from build123d import *

# Parameters (mm, degrees)
F0_R     = 60.254
F0_R_2   = 57.079
F1_DEPTH = 0.854
F2_R     = 60
F3_DEPTH = 0.6


with BuildPart() as f1:
    # F0 (on Top) → F1 (new body, symmetric)
    with BuildSketch(Plane.XY):
        Circle(F0_R)
        Circle(F0_R_2, mode=Mode.SUBTRACT)
    extrude(amount=F1_DEPTH, both=True)

    # F2 (on Top) → F3 (cut, symmetric)
    with BuildSketch(Plane.XY):
        Circle(F2_R)
    extrude(amount=F3_DEPTH, both=True, mode=Mode.SUBTRACT)


solid = f1.part
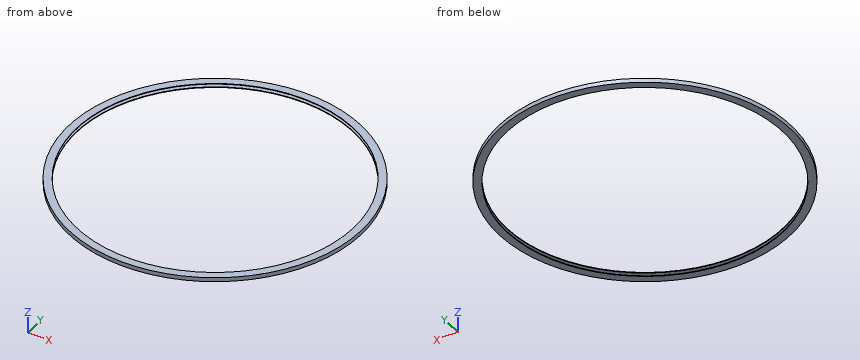
Source: CAD feature listing. Evaluate the final solid. Frame: model axes, mm. Coordinates: 2 decimals unless noted, no trailing zeros. Loops run counter-clockwise (first coordinate to the right, second up) from the corner with the lowest first, then second, coordinate; pieces in that order, holes last. Notation, with made-up numbers: (-8.75, 77.25) - (37.25, 77.25) arc R13 cw to (37.25, 87.25) - close; hole circle Ø3 at (87, 51.25). An arc over 180 degrees is marked (long way). One line per item, written item: value. Start each with the question number.
1. Contact query for a flat-ended pin moving along its axis: P1, Ø12, axis at x = -10.5, y = 46, coming from the +Z side. Output: stop coordinate, or through.
2. Section C-C (z = -0.15). Return the cut outline in (x, y), and give its area (3 significant figures).
3. Ray query, L1, parallel to Y at x = 0, z = -0.65; L2, parallel to Y at x = 0, z = -0.25. Return the intervals inside material, ascending.
4. Section A-A (x = 0). Return the cut outline in (y, z), and give its area (3 significant figures).
Verdict:
1. P1: passes through
2. outline: circle Ø120.51 at (0, 0); hole circle Ø120 at (0, 0)
2. area: 96.0 mm2
3. L1: y = -60.25 to -57.08, 57.08 to 60.25
3. L2: y = -60.25 to -60, 60 to 60.25
4. outline: (-60.25, -0.85) - (-57.08, -0.85) - (-57.08, -0.6) - (-60, -0.6) - (-60, 0.6) - (-57.08, 0.6) - (-57.08, 0.85) - (-60.25, 0.85) - close; (57.08, -0.85) - (60.25, -0.85) - (60.25, 0.85) - (57.08, 0.85) - (57.08, 0.6) - (60, 0.6) - (60, -0.6) - (57.08, -0.6) - close
4. area: 3.84 mm2
